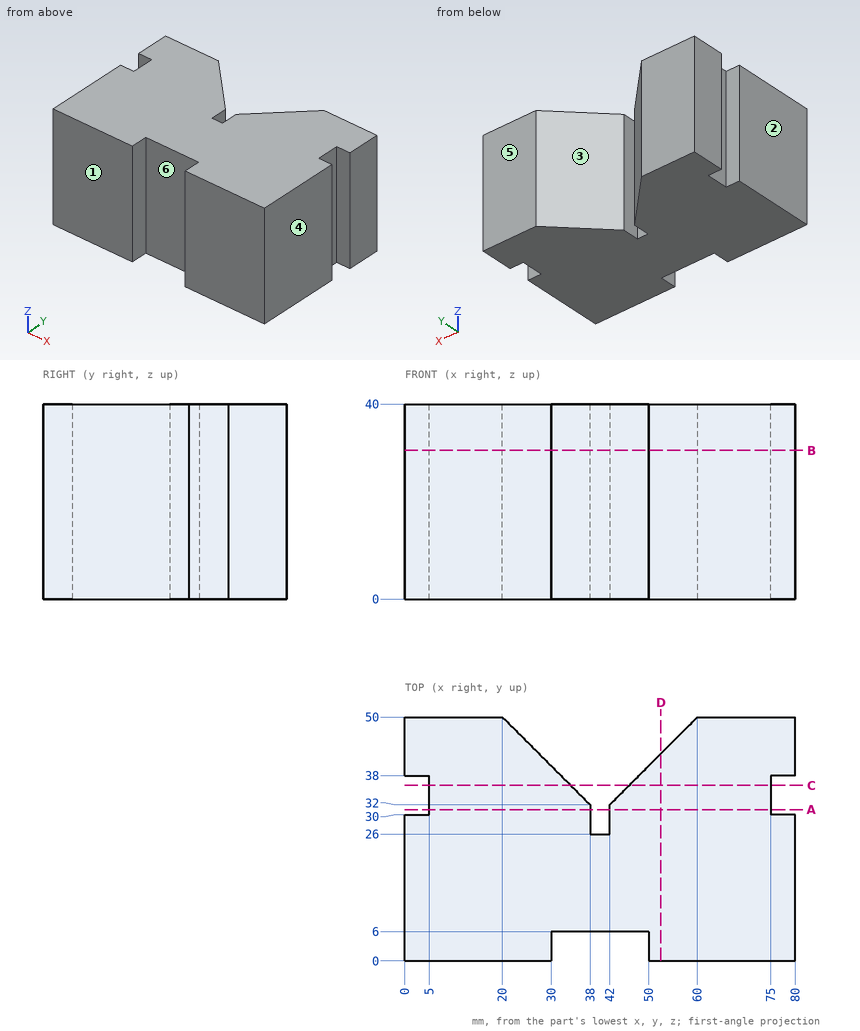
Can you work these out from the drawing? Everything is in mm from the part's minimum corner. A direction names the side the tool comes from. Give positions to 0.01 mm unless a question says otherwise; leave off trailing zeros. Order: outer loops, then holes, each group sorted by start corner. A loop starts at its lowest first (then second) coordinate and runs counter-clockwise, first axis right, second up.
1. For the marked faces 5 and 6, which set-ups out of +Z, -Z, +X, -X, +Y, -Y let a thin tool reach every point of the face, with its end or its side?
2. Suppose I cut it at C-C (y = 36). List the corners of the cut face in (x, z) for me, plus the area to 3 significant figures.
3. Suppose I cut it at B-B (z = 30.5). List the corners of the cut face in (x, y) for me, plus the area to 3 significant figures.
4. Suppose I cut it at A-A (y = 31). List the corners of the cut face in (x, z) for me, plus the area to 3 significant figures.
5. We'd pull the mould along X, two halves only. Please class the marked faces 1, 2, 3 and 4: pulls with the +X half, pulls with the -X half, needs draft (parallel to the pull), parting line crosses it, or undercut.
6. Suppose I cut it at D-D (x = 52.5). List the corners of the cut face in (y, z) for me, plus the area to 3 significant figures.
7. Will these pins go through, and if not, where does the flat tip stop? P1, Ø4, axis at y = 34.5, z = 11.5, coming from the +X side; P2, Ø2.5, axis at y = 32.5, z = 28.5, coming from the -X side; P3, Ø1.2, axis at x = 40, z = 18.5, coming from the +Y side.
8. I need wall thicknesses on L1, parallel to Y at x = 76, z = 29; L2, parallel to X at y = 28, z = 8.5; L3, parallel to X at y = 35, z = 5. Which ranges of each line are inside material? Lowest first, please.
Solved:
1. face 5: +Z, -Z, +X, -X, +Y
1. face 6: +Z, -Z, -Y
2. outline: (5, 0) - (34, 0) - (34, 40) - (5, 40) - close; (46, 0) - (75, 0) - (75, 40) - (46, 40) - close
2. area: 2,320 mm2
3. outline: (0, 0) - (30, 0) - (30, 6) - (50, 6) - (50, 0) - (80, 0) - (80, 30) - (75, 30) - (75, 38) - (80, 38) - (80, 50) - (60, 50) - (42, 32) - (42, 26) - (38, 26) - (38, 32) - (20, 50) - (0, 50) - (0, 38) - (5, 38) - (5, 30) - (0, 30) - close
3. area: 3,380 mm2
4. outline: (5, 0) - (38, 0) - (38, 40) - (5, 40) - close; (42, 0) - (75, 0) - (75, 40) - (42, 40) - close
4. area: 2,640 mm2
5. face 1: needs draft
5. face 2: pulls with the -X half
5. face 3: undercut
5. face 4: pulls with the +X half
6. outline: (0, 0) - (42.5, 0) - (42.5, 40) - (0, 40) - close
6. area: 1,700 mm2
7. P1: stops at x = 75
7. P2: stops at x = 5
7. P3: stops at y = 26
8. L1: y = 0 to 30, 38 to 50
8. L2: x = 0 to 38, 42 to 80
8. L3: x = 5 to 35, 45 to 75
